```python
from build123d import *

# Parameters (mm, degrees)
F2_T     = 1
F3_R     = 5.5
F4_DEPTH = 20.001


with BuildPart() as f1:
    # F0 (on Front) → F1 (revolve)
    with BuildSketch(Plane.XZ):
        with BuildLine():
            Line((0, 19), (0, -19))
            Line((0, -19), (100, -19))
            ThreePointArc((100, -19), (53.4883164813, 9.1797802139), (0, 19))
        make_face()
    revolve(axis=Axis((0, 0, 0), (0, 0, -1)))

    # F2
    f2_openings = [f1.faces().sort_by_distance(p)[0] for p in [
        (0, 0, -19),
    ]]
    offset(amount=F2_T, openings=f2_openings)

    # F3 (on Top) → F4 (cut, through all)
    with BuildSketch(Plane.XY):
        Circle(F3_R)
    extrude(amount=F4_DEPTH, mode=Mode.SUBTRACT)


solid = f1.part
```
Work out the finished part from the listing and answer in its coordinate system (mm). Coordinates: 2 decimals unless noted, no trailing zeros. Write each loop counter-clockwise with the first axis right and the second up, starting at its lowest first coordinate (ties: lowest second). Pieces come first, ordered by that corner, then holes.
Q1. Find the intervals of material crossed by line 1 (X direction, y = 0, z = -4.5); line 2 (Y direction, x = 39, z = -1); line 3 (Y direction, x = 17.5, z = -4.5), in increasing order.
Q2. Each of these flat-tipped pins is pushed along its axis until it touches: pin 1 Ø1.5 at (x, y) = (43, -24) entering from -Z; pin 2 Ø6 at (x, y) = (-36.5, 38) entering from -Z; pin 3 Ø1.5 at (x, z) = (-57, -6) entering from +Y. Where does it stop, or does it pass through?
Q3. Determine the mould class of faces 1 (the face through (-75, 67, -19)), 2 (the face through (-1.19, -5.37, 19.39)) for opening direction Y: released by +Y, released by -Y, zero draft, split by the parting line, or undercut.
Q4. A cutting plane is placed at A-A, the plane y = 0. Give the vertices of the cut face in (x, z), then the cut area to 3 significant figures.
Q5. A cutting plane is placed at C-C, the plane z = -16. Give the vertices of the cut face in (x, y).
Q6. A cutting plane is placed at D-D, the plane y = -27.5. Give the vertices of the cut face in (x, z), then the cut area to 3 significant figures.
Findings below:
1. line 1: x = -82.63 to -80.78, 80.78 to 82.63
1. line 2: y = -66.37 to -64.05, 64.05 to 66.37
1. line 3: y = -80.75 to -78.86, 78.86 to 80.75
2. pin 1: stops at z = 10.46
2. pin 2: stops at z = 8.32
2. pin 3: stops at y = 64.52
3. face 1: zero draft
3. face 2: undercut
4. outline: (-101.5, -19) - (-100, -19) arc R150.58 cw to (-5.5, 18.9) - (-5.5, 19.9) arc R151.58 ccw to start; (5.5, 18.9) arc R150.58 cw to (100, -19) - (101.5, -19) arc R151.58 ccw to (5.5, 19.9) - close
4. area: 210 mm2
5. outline: circle Ø196.14 at (0, 0); hole circle Ø193.03 at (0, 0)
6. outline: (-97.7, -19) - (-96.14, -19) arc R148.05 cw to (96.14, -19) - (97.7, -19) arc R149.06 ccw to start
6. area: 215 mm2
